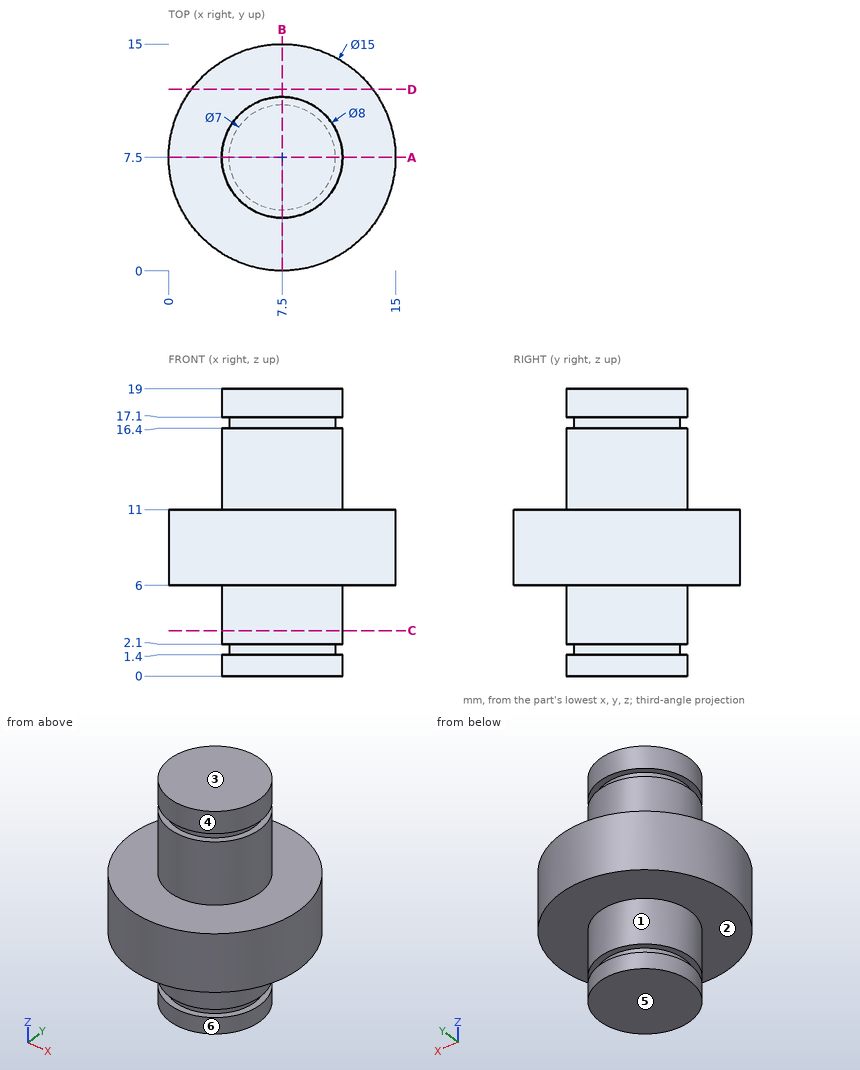
Could you check a few things on this drawing? It's one solid part, dimensions in mm from its lowest x, y, z. A direction names the side the tool comes from. Round coordinates to 2 decimals unless told otherwise and drop trailing zeros. Loops run counter-clockwise (first coordinate to the right, second up) from the corner with the lowest first, then second, coordinate; pieces in that order, holes last. Notation, with made-up numbers: M -18.75,-35.5 L 30.25,-35.5 A13 ccw 30.25,-21.5 Z; hole C 14,-21.5 d8. An arc over 180 degrees is marked long. Write item = value, one per line. Start each with the question number.
(1) Suppose I cut it at D-D on y = 12. Write out the boundary of the cut face in (x, z), plus the area to 3 significant figures.
(2) I'm going to push flat-ended pins straight in: P1, Ø1, axis at y = 5, z = 15.5, coming from the -X side; P2, Ø3, axis at y = 3.5, z = 16, coming from the -X side; P3, Ø1.5, axis at x = 2.5, z = 8.5, coming from the -Y side. Where does each tip first touch, or does it pass through?
(3) Suppose I cut it at A-A on y = 7.5. Write out the boundary of the cut face in (x, z), plus the area to 3 significant figures.
(4) Suppose I cut it at C-C on z = 3. Write out the boundary of the cut face in (x, y).
(5) Which directions (+Z, -Z, +X, -X, +Y, -Y) give clear straight access to the entire face, cutting with the end or side of a thin tool? Please do the marked faces 4, 5 and 6.
(6) If we mould it in two halves opening along Z, with no side actions, what happens to the marked faces 1, 2 and 3? For each: released by +Z, released by -Z, zero draft, split by the parting line, or undercut.
(7) I need wall thicknesses on line 1 along Z through (x, y) = (4, 9); line 2 along Z through (x, y) = (1, 4); line 3 along X through (y, z) = (2.5, 9). Which ranges of each line are inside material? Lowest first, please.
Answer block:
q1.outline = M 1.5,6 L 13.5,6 L 13.5,11 L 1.5,11 Z
q1.area = 60.0 mm²
q2.P1 = 4.04
q2.P2 = 4.38
q2.P3 = 1.32
q3.outline = M 0,6 L 3.5,6 L 3.5,2.1 L 4,2.1 L 4,1.4 L 3.5,1.4 L 3.5,0 L 11.5,0 L 11.5,1.4 L 11,1.4 L 11,2.1 L 11.5,2.1 L 11.5,6 L 15,6 L 15,11 L 11.5,11 L 11.5,16.4 L 11,16.4 L 11,17.1 L 11.5,17.1 L 11.5,19 L 3.5,19 L 3.5,17.1 L 4,17.1 L 4,16.4 L 3.5,16.4 L 3.5,11 L 0,11 Z
q3.area = 186 mm²
q4.outline = C 7.5,7.5 d8
q5.face_4 = +Z
q5.face_5 = -Z, +X, -X, +Y, -Y
q5.face_6 = -Z
q6.face_1 = zero draft
q6.face_2 = released by -Z
q6.face_3 = released by +Z
q7.line_1 = 0 to 1.4, 2.1 to 16.4, 17.1 to 19
q7.line_2 = 6 to 11
q7.line_3 = 1.91 to 13.09
